Input: part model. Units: mm. Frame: model coordinates. Face numbers are marked on the shaded views. A direction names the side the tool comes from. Coordinates: 2 decimals unless noted, no trailing zeros. Order: outer loops, then holes, each group sorted by start corner. A loop starts at its lowest first (then second) coordinate and runs counter-clockwise, first axis right, second up. Notation, with made-up numbers: M -13,30 L 4,30 A18 cw 4,34 Z; hole C 70,24 d8. An arc over 180 degrees is marked long. One line per item, written item: value.
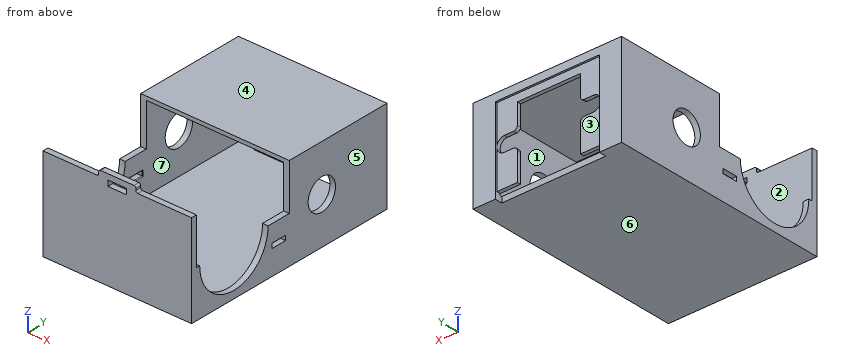
```python
from build123d import *

# Parameters (mm, degrees)
SKETCH_1_W           = 40
SKETCH_1_H           = 60
EXTRUDE_1_DEPTH      = 25
SHELL_1_T            = -1.5
SKETCH_2_R           = 10.5
CUT_EXTRUDE_1_DEPTH  = 75
SKETCH_3_W           = 40
SKETCH_3_H           = 30
EXTRUDE_2_DEPTH      = 1
SKETCH_4_W           = 40
SKETCH_4_H           = 28.5
CUT_EXTRUDE_2_DEPTH  = 12.5
SKETCH_5_R           = 4.2
CUT_EXTRUDE_3_DEPTH  = 1.5
SKETCH_6_W           = 28
SKETCH_6_H           = 26
CUT_EXTRUDE_4_DEPTH  = 0.5
CUT_EXTRUDE_7_DEPTH  = 3.5
SKETCH_9_W           = 28
SKETCH_9_H           = 2
CUT_EXTRUDE_8_DEPTH  = 0.5
FILLET_1_R           = 1
CUT_EXTRUDE_9_DEPTH  = 1.5
SKETCH_18_W          = 10
SKETCH_18_H          = 1.5
EXTRUDE_6_DEPTH      = 1.5
SKETCH_22_W          = 5
SKETCH_22_H          = 1.5
CUT_EXTRUDE_13_DEPTH = 2
FILLET_4_R           = 0.5
SKETCH_26_W          = 1.25
SKETCH_26_H          = 4.2
CUT_EXTRUDE_15_DEPTH = 41
FILLET_5_R           = 0.2
SKETCH_17_R          = 4.2
CUT_EXTRUDE_16_DEPTH = 41
EXTRUDE_START        = 1.5
EXTRUDE_9_DEPTH      = 1.5


with BuildPart() as part:
    # 草图1 → 凸台-拉伸1 (new body)
    with BuildSketch(Plane.XY):
        Rectangle(SKETCH_1_W, SKETCH_1_H)
    extrude(amount=EXTRUDE_1_DEPTH)

    # 抽壳1
    shell_1_openings = [part.faces().sort_by_distance(p)[0] for p in [
        (0, 0, 25),
    ]]
    offset(amount=SHELL_1_T, openings=shell_1_openings, kind=Kind.INTERSECTION)

    # 草图2 → 切除-拉伸1 (cut)
    with BuildSketch(Plane(origin=(20, 0, 0), x_dir=(0, 0, -1), z_dir=(1, 0, 0))):
        with Locations((-12.5, -17)):
            Circle(SKETCH_2_R)
    extrude(amount=-CUT_EXTRUDE_1_DEPTH, mode=Mode.SUBTRACT)

    # 草图3 → 凸台-拉伸2 (add)
    with BuildSketch(Plane.XY.offset(25)):
        with Locations((0, 15)):
            Rectangle(SKETCH_3_W, SKETCH_3_H)
    extrude(amount=-EXTRUDE_2_DEPTH)

    # 草图4 → 切除-拉伸2 (cut)
    with BuildSketch(Plane.XY.offset(25)):
        with Locations((0, -14.25)):
            Rectangle(SKETCH_4_W, SKETCH_4_H)
    extrude(amount=-CUT_EXTRUDE_2_DEPTH, mode=Mode.SUBTRACT)

    # 草图5 → 切除-拉伸3 (cut)
    with BuildSketch(Plane(origin=(0, 30, 0), x_dir=(1, 0, 0), z_dir=(0, 1, 0))):
        with Locations((-20, -12.5)):
            Circle(SKETCH_5_R)
        with Locations((20, -12.5)):
            Circle(SKETCH_5_R)
    extrude(amount=-CUT_EXTRUDE_3_DEPTH, mode=Mode.SUBTRACT)

    # 草图6 → 切除-拉伸4 (cut)
    with BuildSketch(Plane(origin=(0, 30, 0), x_dir=(1, 0, 0), z_dir=(0, 1, 0))):
        with Locations((0, -8)):
            Rectangle(SKETCH_6_W, SKETCH_6_H)
    extrude(amount=-CUT_EXTRUDE_4_DEPTH, mode=Mode.SUBTRACT)

    # 草图8 → 切除-拉伸7 (cut)
    with BuildSketch(Plane(origin=(0, 29.5, 0), x_dir=(1, 0, 0), z_dir=(0, 1, 0))):
        with BuildLine():
            Line((-8.5, -4), (8.5, -4))
            Line((8.5, -4), (8.5, -10.5))
            Line((8.5, -10.5), (12, -10.5))
            ThreePointArc((12, -10.5), (14, -12.5), (12, -14.5))
            Line((12, -14.5), (8.5, -14.5))
            Line((8.5, -14.5), (8.5, -21))
            Line((8.5, -21), (-8.5, -21))
            Line((-8.5, -21), (-8.5, -14.5))
            Line((-8.5, -14.5), (-12, -14.5))
            ThreePointArc((-12, -14.5), (-14, -12.5), (-12, -10.5))
            Line((-12, -10.5), (-8.5, -10.5))
            Line((-8.5, -10.5), (-8.5, -4))
        make_face()
    extrude(amount=-CUT_EXTRUDE_7_DEPTH, mode=Mode.SUBTRACT)

    # 草图9 → 切除-拉伸8 (cut)
    with BuildSketch(Plane(origin=(0, 30, 0), x_dir=(1, 0, 0), z_dir=(0, 1, 0))):
        with Locations((0, -22)):
            Rectangle(SKETCH_9_W, SKETCH_9_H)
    extrude(amount=-CUT_EXTRUDE_8_DEPTH, mode=Mode.SUBTRACT)

    # 圆角1
    fillet_1_edges = [part.edges().sort_by_distance(p)[0] for p in [
        (8.5, 29, 14.5),
        (-8.5, 29, 14.5),
        (-8.5, 29, 10.5),
        (8.5, 29, 10.5),
    ]]
    fillet(fillet_1_edges, radius=FILLET_1_R)

    # 草图10 → 切除-拉伸9 (cut)
    with BuildSketch(Plane(origin=(0, 29.5, 0), x_dir=(1, 0, 0), z_dir=(0, 1, 0))):
        Polygon((8.5, -4), (8.5, -2), (14, -2), (14, 0), (8.5, 0), (-8.5, 0), (-14, 0), (-14, -2), (-8.5, -2), (-8.5, -4), align=None)
    extrude(amount=-CUT_EXTRUDE_9_DEPTH, mode=Mode.SUBTRACT)

    # 草图18 → 凸台-拉伸6 (add)
    with BuildSketch(Plane.XY.offset(25)):
        with Locations((0, -29.25)):
            Rectangle(SKETCH_18_W, SKETCH_18_H)
    extrude(amount=EXTRUDE_6_DEPTH)

    # 草图22 → 切除-拉伸13 (cut)
    with BuildSketch(Plane(origin=(0, -28.5, 0), x_dir=(1, 0, 0), z_dir=(0, 1, 0))):
        with Locations((0, -24.25)):
            Rectangle(SKETCH_22_W, SKETCH_22_H)
    extrude(amount=-CUT_EXTRUDE_13_DEPTH, mode=Mode.SUBTRACT)

    # 圆角4
    fillet_4_edges = [part.edges().sort_by_distance(p)[0] for p in [
        (5, -29.25, 25),
        (-5, -29.25, 25),
        (5, -29.25, 26.5),
        (-5, -29.25, 26.5),
    ]]
    fillet(fillet_4_edges, radius=FILLET_4_R)

    # 草图26 → 切除-拉伸15 (cut)
    with BuildSketch(Plane(origin=(20, 0, 0), x_dir=(0, 0, -1), z_dir=(1, 0, 0))):
        with Locations((-7.25, -3.25)):
            Rectangle(SKETCH_26_W, SKETCH_26_H)
    extrude(amount=-CUT_EXTRUDE_15_DEPTH, mode=Mode.SUBTRACT)

    # 圆角5
    fillet_5_edges = [part.edges().sort_by_distance(p)[0] for p in [
        (-18.5, -1.15, 7.25),
        (-18.5, -3.25, 7.875),
        (-18.5, -5.35, 7.25),
        (-18.5, -3.25, 6.625),
        (18.5, -3.25, 6.625),
        (18.5, -5.35, 7.25),
        (18.5, -3.25, 7.875),
        (18.5, -1.15, 7.25),
    ]]
    fillet(fillet_5_edges, radius=FILLET_5_R)

    # 草图17 → 切除-拉伸16 (cut)
    with BuildSketch(Plane(origin=(20, 0, 0), x_dir=(0, 0, -1), z_dir=(1, 0, 0))):
        with Locations((-12.5, 10)):
            Circle(SKETCH_17_R)
    extrude(amount=-CUT_EXTRUDE_16_DEPTH, mode=Mode.SUBTRACT)

    # 草图27 → 凸台-拉伸9 (add)
    with BuildSketch(Plane(origin=(0, 28.5, 0), x_dir=(1, 0, 0), z_dir=(0, 1, 0)).offset(EXTRUDE_START)):
        with BuildLine():
            Line((-20, -8.3), (-20, -16.7))
            ThreePointArc((-20, -16.7), (-15.8, -12.5), (-20, -8.3))
        make_face()
        with BuildLine():
            Line((20, -8.3), (20, -16.7))
            ThreePointArc((20, -16.7), (15.8, -12.5), (20, -8.3))
        make_face()
    extrude(amount=-EXTRUDE_9_DEPTH)


solid = part.part
```
(1) Cut plane C-C on z = 22. Output: boundary loops of the cut face in (x, y).
Data:
outline: M -20,-30 L 20,-30 L 20,-28.5 L -20,-28.5 Z; M -20,0 L -18.5,0 L -18.5,28.5 L 18.5,28.5 L 18.5,0 L 20,0 L 20,30 L 14,30 L 14,29.5 L -14,29.5 L -14,30 L -20,30 Z
(2) Cut plane B-B on x = -1.5. Output: boundary loops of the cut face in (y, z), plus the area to 3 significant figures.
Data:
outline: M -30,0 L 28,0 L 28,1.5 L -28.5,1.5 L -28.5,23.5 L -30,23.5 Z; M -30,25 L -28.5,25 L -28.5,26.5 L -30,26.5 Z; M 0,24 L 28.5,24 L 28.5,21 L 29.5,21 L 29.5,23 L 30,23 L 30,25 L 0,25 Z
area: 156 mm2
(3) Access query for the marked faces 1, 2, 3 and 4. Directions: +Z, -Z, +X, -X, +Y, -Y. A direction counts if a zero-diameter tool reaches every point of the face in a straight line with its end or side. Return the directions, or none.
Data:
face 1: none
face 2: +Z
face 3: -Z, +Y
face 4: +Z, +X, -X, +Y
(4) Draft query along X for the marked faces 5, 6 and 7. Return one class per face: released by +X, released by -X, zero draft, split by the parting line, or undercut.
Data:
face 5: released by +X
face 6: zero draft
face 7: undercut
(5) First-contact query: pin 1 (10 mm diameter, centred on y = -17.5, z = 5, fed in from -X); pin 2 (8 mm diameter, centred on x = 2, z = 5, fed in from +Y); pin 3 (2 mm diameter, centred on x = -4.5, z = 18.5, fed in from +Y); pin 4 (5 mm diameter, centred on y = 10, z = 12.5, fed in from -X). Flat tips, straight axial feed; report the tip coordinate or a pass-through.
Data:
pin 1: stops at x = -20
pin 2: stops at y = 28
pin 3: stops at y = -28.5
pin 4: passes through
(6) Ray query, line 1 (X direction, y = 22, z = 3); line 2 (Z direction, x = 14, y = 23); line 3 (Y direction, x = 12, z = 9.5). Return the intervals inside material, ascending. Write a range as from..to.
Data:
line 1: x = -20..-18.5, 18.5..20
line 2: z = 0..1.5, 24..25
line 3: y = -30..-28.5, 28.5..29.5
(7) Cut plane A-A on y = 10. Output: boundary loops of the cut face in (x, z), plus the area to 3 significant figures.
Data:
outline: M -20,0 L 20,0 L 20,8.3 L 18.5,8.3 L 18.5,1.5 L -18.5,1.5 L -18.5,8.3 L -20,8.3 Z; M -20,16.7 L -18.5,16.7 L -18.5,24 L 18.5,24 L 18.5,16.7 L 20,16.7 L 20,25 L -20,25 Z
area: 142 mm2
(8) Cut plane D-D on y = 25.5. Output: boundary loops of the cut face in (x, z), plus the area to 4 significant figures.
Data:
outline: M -20,0 L 20,0 L 20,25 L -20,25 Z; hole M -18.5,1.5 L 18.5,1.5 L 18.5,24 L -18.5,24 Z
area: 167.5 mm2
